Autodesk Inventor part; units mm, degrees
ref_plane "YZ Plane" through (0, 0, 0) normal (1, 0, 0) x (0, 1, 0)
ref_plane "XZ Plane" through (0, 0, 0) normal (0, 1, 0) x (-1, 0, 0)
ref_plane "XY Plane" through (0, 0, 0) normal (0, 0, 1) x (1, 0, 0)
sketch "Sketch1" plane through (0, 0, 0) normal (1, 0, 0) x (0, 1, 0)
  line L0 (10.4573, 9.6454) -> (-548.3427, 9.6454)
  line L1 (-548.3427, 9.6454) -> (-548.3427, -53.8546)
  line L2 (-548.3427, -53.8546) -> (10.4573, -53.8546)
  line L3 (10.4573, -53.8546) -> (10.4573, 9.6454)
  point P0 (0, 0)
  dimension "d0" = 558.8
  dimension "d1" = 63.5
extrude "Extrusion1" add sketch "Sketch1" along normal blind 19.05
sketch "Sketch2" plane through (19.05, 0, 0) normal (1, 0, 0) x (0, 0, -1)
  line L0 (-4.0419, -15.157) -> (46.7581, -15.157)
  line L1 (46.7581, -15.157) -> (46.7581, -91.357)
  line L2 (46.7581, -91.357) -> (-4.0419, -91.357)
  line L3 (-4.0419, -91.357) -> (-4.0419, -15.157)
  point P0 (0, 0)
  dimension "d4" = 50.8
  dimension "d5" = 76.2
extrude "Extrusion2" cut sketch "Sketch2" against normal blind 19.05
properties part number "blade" material "Rubber, Silicone"
Check sheet for the modelled part. Datum: model origin and axes. Units: mm. A direction names the side the tool comes from. Coordinates: 2 decimals unless noted, no trailing zeros. Write each loop counter-clockwise with the first axis right and the second up, starting at its lowest first coordinate (ties: lowest second). Pieces come first, ordered by that corner, then holes. Notation, with made-up numbers: (-1.5, -37) - (47.5, -37) arc R8 cw to (47.5, -22) - close; hole circle Ø2 at (16, 56). An arc over 180 degrees is marked (long way). One line per question, with ' | ' between items.
Item 1: Sectioned sample at C-C on z = -9.5. Record the boundary of the cut face in (x, y), plus the area to 3 significant figures.
Determined:
outline: (0, -548.34) - (19.05, -548.34) - (19.05, -91.36) - (0, -91.36) - close; (0, -15.16) - (19.05, -15.16) - (19.05, 10.46) - (0, 10.46) - close | area: 9,190 mm2
Item 2: Sectioned sample at A-A on x = 7.25. Record the boundary of the cut face in (y, z), plus the area to 3 significant figures.
Determined:
outline: (-548.34, -53.85) - (10.46, -53.85) - (10.46, 9.65) - (-548.34, 9.65) - close; hole (-91.36, -46.76) - (-15.16, -46.76) - (-15.16, 4.04) - (-91.36, 4.04) - close | area: 31,600 mm2
Item 3: Access from +Z, -Z, +X, -X, +Y, -Y to the whole of each face (thin tool, end or side, straight path). Record for faces 1 (the face through (10, -91.357, -22)), 2 (the face through (9, -265, 9.645)).
Determined:
face 1: +X, -X | face 2: +Z, +X, -X, +Y, -Y
Item 4: Thickness scan on line 1 (Y direction, x = 18.25, z = -39). Record the ranges inside material, lowest first. Write a range as [from, to].
Determined:
line 1: y = [-548.34, -91.36], [-15.16, 10.46]
Item 5: Sectioned sample at B-B on y = -49.5. Record the boundary of the cut face in (x, z).
Determined:
outline: (0, -53.85) - (19.05, -53.85) - (19.05, -46.76) - (0, -46.76) - close; (0, 4.04) - (19.05, 4.04) - (19.05, 9.65) - (0, 9.65) - close
Item 6: Gauge pin test, flat end, axial feed: P1, Ø10, axis at y = -464.5, z = -33, coming from the -X side. Record the tip position at first contact, or that the pin passes through.
Determined:
P1: stops at x = 0
Item 7: Mould release check, pull along Y, two halves, no side actions. Record for faces 3 (the face through (10, -54, 4.042)), 4 (the face through (10, -15.157, -21)), 5 (the face through (0, -335, -22)), 6 (the face through (9, 10.457, -23)): pulls with the +Y half, pulls with the -Y half, needs draft (parallel to the pull), parting line crosses it, or undercut.
Determined:
face 3: undercut | face 4: undercut | face 5: needs draft | face 6: pulls with the +Y half
